from build123d import *

# Parameters (mm, degrees)
SKETCH_1_W          = 28.5
SKETCH_1_H          = 20
SKETCH_1_R          = 2.055
EXTRUDE_1_DEPTH     = 4.5
CHAMFER_1_SIZE      = 2.5
CHAMFER_2_SIZE      = 0.445
SKETCH_2_R          = 15
CUT_EXTRUDE_1_DEPTH = 5.5


with BuildPart() as part:
    # Эскиз1 → Бобышка-Вытянуть1 (new body)
    with BuildSketch(Plane.XY):
        Rectangle(SKETCH_1_W, SKETCH_1_H)
        with Locations((9.25, 5)):
            Circle(SKETCH_1_R, mode=Mode.SUBTRACT)
    extrude(amount=EXTRUDE_1_DEPTH)

    # Фаска1
    chamfer_1_edges = [part.edges().sort_by_distance(p)[0] for p in [
        (14.25, 10, 2.25),
    ]]
    chamfer(chamfer_1_edges, length=CHAMFER_1_SIZE)

    # Фаска2
    chamfer_2_edges = [part.edges().sort_by_distance(p)[0] for p in [
        (7.195, 5, 0),
        (7.195, 5, 4.5),
    ]]
    chamfer(chamfer_2_edges, length=CHAMFER_2_SIZE)

    # Зеркальное отражение1: part across plane


with BuildPart() as part_1:
    add(part.part)
    add(part.part.mirror(Plane(origin=(-14.25, -10, 4.5), x_dir=(0, 0, 1), z_dir=(0, 1, 0))))

    # Зеркальное отражение2: part across plane


with BuildPart() as part_2:
    add(part_1.part)
    add(part_1.part.mirror(Plane(origin=(-14.25, -10, 4.5), x_dir=(0, 0, 1), z_dir=(1, 0, 0))))

    # Эскиз2 → Вырез-Вытянуть1 (cut, through all)
    with BuildSketch(Plane.XY.offset(4.5)):
        with Locations((-14.25, -10)):
            Circle(SKETCH_2_R)
    extrude(amount=-CUT_EXTRUDE_1_DEPTH, mode=Mode.SUBTRACT)


solid = part_2.part
Source: CAD feature listing. Evaluate the final solid. Frame: model axes, mm. Give positions to 0.01 mm unless a question says otherwise; leave off trailing zeros. Loops run counter-clockwise (first coordinate to the right, second up) from the corner with the lowest first, then second, coordinate; pieces in that order, holes last. Notation, with made-up numbers: (38, 47.25) -> (75, 47.25) arc R19 cw to (75, 74.25) -> close; hole circle Ø3 at (46.5, 0). An arc over 180 degrees is marked (long way). Use a Markdown table: item, result. Add a question column.
1) Section query B-B, the plane x = 9.25. Return the cut outline in (y, z) (3 decimals), then the cut area to 3 significant figures.
2) Line query: line 1 along Y through (x, z) = (9.25, 2.1) (3 decimals); line 2 along X through (y, z) = (-26.5, 1.2); line 3 along Y through (x, z) = (-37, 3.7). Output: solid intervals per line, ascending. Write a range as [from, to].
3) Section query C-C, the plane z = 3. Return the cut outline in (x, y) (3 decimals), then the cut area to 3 significant figures.
4) Section query D-D, the plane x = -15. Return the cut outline in (y, z), then the cut area to 3 significant figures.
5) Section query A-A, the plane y = -10. Return the cut outline in (x, z).
Numbers:
| question | item | result |
|---|---|---|
| 1 | outline | (-30, 0) -> (-27.5, 0) -> (-27.055, 0.445) -> (-27.055, 4.055) -> (-27.5, 4.5) -> (-30, 4.5) -> close; (-22.945, 0.445) -> (-22.5, 0) -> (2.5, 0) -> (2.945, 0.445) -> (2.945, 4.055) -> (2.5, 4.5) -> (-22.5, 4.5) -> (-22.945, 4.055) -> close; (7.055, 0.445) -> (7.5, 0) -> (10, 0) -> (10, 4.5) -> (7.5, 4.5) -> (7.055, 4.055) -> close |
| 1 | area | 142 mm2 |
| 2 | line 1 | y = [-30, -27.055], [-22.945, 2.945], [7.055, 10] |
| 2 | line 2 | x = [-42.75, -39.15], [-36.35, 7.85], [10.65, 14.25] |
| 2 | line 3 | y = [-30, -26.91], [-23.09, 3.09], [6.91, 10] |
| 3 | outline | (-42.75, -27.5) -> (-40.25, -30) -> (11.75, -30) -> (14.25, -27.5) -> (14.25, 7.5) -> (11.75, 10) -> (-40.25, 10) -> (-42.75, 7.5) -> close; hole circle Ø4.11 at (-37.75, -25); hole circle Ø4.11 at (-37.75, 5); hole circle Ø30 at (-14.25, -10); hole circle Ø4.11 at (9.25, -25); hole circle Ø4.11 at (9.25, 5) |
| 3 | area | 1,510 mm2 |
| 4 | outline | (-30, 0) -> (-24.98, 0) -> (-24.98, 4.5) -> (-30, 4.5) -> close; (4.98, 0) -> (10, 0) -> (10, 4.5) -> (4.98, 4.5) -> close |
| 4 | area | 45.2 mm2 |
| 5 | outline | (-42.75, 0) -> (-29.25, 0) -> (-29.25, 4.5) -> (-42.75, 4.5) -> close; (0.75, 0) -> (14.25, 0) -> (14.25, 4.5) -> (0.75, 4.5) -> close |
